Check sheet for the modelled part. Datum: model origin and axes. Units: mm. Face numbers are marked on the shaded views. A direction names the side the tool comes from. Round coordinates to 2 decimals unless told otherwise and drop trailing zeros. Loops run counter-clockwise (first coordinate to the right, second up) from the corner with the lowest first, then second, coordinate; pieces in that order, holes last. Notation, with made-up numbers: (18, 25.5) -> (32, 25.5) arc R3 ccw to (32, 29.5) -> close; hole circle Ø5 at (-10, 3). An arc over 180 degrees is marked (long way). One line per question, with ' | ' between items.
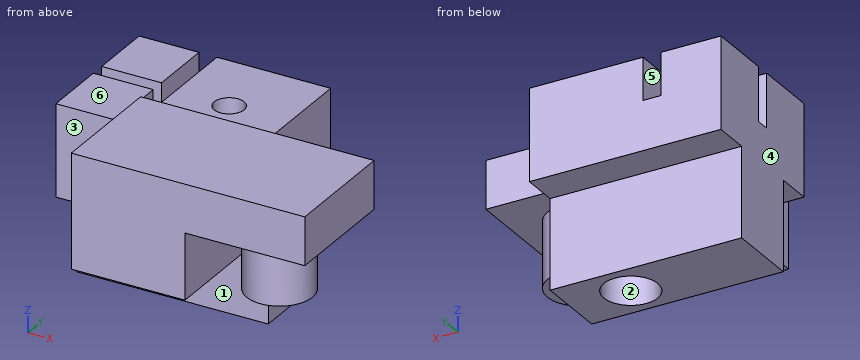
```python
from build123d import *

# Parameters (mm, degrees)
SKETCH_1_W          = 16
SKETCH_1_H          = 12
EXTRUDE_1_DEPTH     = 7.65
SKETCH_2_W          = 5
SKETCH_2_H          = 1.2
CUT_EXTRUDE_1_DEPTH = 4.5
SKETCH_3_R          = 7.15
CUT_EXTRUDE_2_DEPTH = 1.5
SKETCH_4_W          = 16
SKETCH_4_H          = 6
EXTRUDE_2_DEPTH     = 7.5
SKETCH_5_R          = 2.25
CUT_EXTRUDE_3_DEPTH = 7.5
SKETCH_6_R          = 1.25
CUT_EXTRUDE_4_DEPTH = 8.65
SKETCH_7_W          = 9.5
SKETCH_7_H          = 7.65
EXTRUDE_3_DEPTH     = 9
EXTRUDE_START       = -9.5
SKETCH_8_W          = 4
SKETCH_8_H          = 10
EXTRUDE_4_DEPTH     = 19.5
SKETCH_9_R          = 2.75
EXTRUDE_5_DEPTH     = 5.5


with BuildPart() as part:
    # Эскиз1 → Бобышка-Вытянуть1 (new body)
    with BuildSketch(Plane.XY):
        with Locations((-13.599693696, 25)):
            Rectangle(SKETCH_1_W, SKETCH_1_H)
    extrude(amount=EXTRUDE_1_DEPTH)

    # Эскиз2 → Вырез-Вытянуть1 (cut)
    with BuildSketch(Plane.XY.offset(7.65)):
        with Locations((-19.099693696, 25)):
            Rectangle(SKETCH_2_W, SKETCH_2_H)
    extrude(amount=-CUT_EXTRUDE_1_DEPTH, mode=Mode.SUBTRACT)

    # Эскиз3 → Вырез-Вытянуть2 (cut)
    with BuildSketch(Plane.ZY.offset(16.599693696)):
        with Locations((8, 25)):
            Circle(SKETCH_3_R)
    extrude(amount=-CUT_EXTRUDE_2_DEPTH, mode=Mode.SUBTRACT)

    # Эскиз4 → Бобышка-Вытянуть2 (add)
    with BuildSketch(Plane(origin=(0, 0, 0), x_dir=(-1, 0, 0), z_dir=(0, 0, -1))):
        with Locations((13.599693696, 25)):
            Rectangle(SKETCH_4_W, SKETCH_4_H)
    extrude(amount=EXTRUDE_2_DEPTH)

    # Эскиз5 → Вырез-Вытянуть3 (cut)
    with BuildSketch(Plane(origin=(0, 0, -7.5), x_dir=(-1, 0, 0), z_dir=(0, 0, -1))):
        with Locations((10.599693696, 25)):
            Circle(SKETCH_5_R)
    extrude(amount=-CUT_EXTRUDE_3_DEPTH, mode=Mode.SUBTRACT)

    # Эскиз6 → Вырез-Вытянуть4 (cut, through all)
    with BuildSketch(Plane(origin=(0, 0, 0), x_dir=(-1, 0, 0), z_dir=(0, 0, -1))):
        with Locations((10.599693696, 25)):
            Circle(SKETCH_6_R)
    extrude(amount=-CUT_EXTRUDE_4_DEPTH, mode=Mode.SUBTRACT)

    # Эскиз7 → Бобышка-Вытянуть3 (add)
    with BuildSketch(Plane.XZ.offset(-19)):
        with Locations((-10.349693696, 3.825)):
            Rectangle(SKETCH_7_W, SKETCH_7_H)
    extrude(amount=EXTRUDE_3_DEPTH)

    # Эскиз8 → Бобышка-Вытянуть4 (add)
    with BuildSketch(Plane(origin=(-5.599693696, 0, 0), x_dir=(0, 0, -1), z_dir=(1, 0, 0)).offset(EXTRUDE_START)):
        with Locations((-7.5, 15)):
            Rectangle(SKETCH_8_W, SKETCH_8_H)
    extrude(amount=EXTRUDE_4_DEPTH)

    # Эскиз9 → Бобышка-Вытянуть5 (add)
    with BuildSketch(Plane(origin=(0, 0, 5.5), x_dir=(-1, 0, 0), z_dir=(0, 0, -1))):
        with Locations((0.599693696, 15)):
            Circle(SKETCH_9_R)
    extrude(amount=EXTRUDE_5_DEPTH)


solid = part.part
```
(1) Sectioned sample at B-B, the plane z = 0.5. Record the cut outline in (x, y), and give its area (3 significant figures).
Answer:
outline: (-21.6, 19) -> (-15.1, 19) -> (-15.1, 10) -> (-5.6, 10) -> (-5.6, 31) -> (-21.6, 31) -> close; circle Ø5.5 at (-0.6, 15); hole circle Ø2.5 at (-10.6, 25) | area: 296 mm2
(2) Set-up check for the marked faces 1, 2 and 3: record each of +Z, -Z, +X, -X, +Y, -Y from which the full face is reachable in a straight line by a thin tool's end or side.
Answer:
face 1: -Z, +X, -X, -Y | face 2: -Z | face 3: +Z, -Z, -X, -Y
(3) Go/stop test with flat-tipped pins: pin 1 (3 mm diameter, centred on x = -16, y = 25, fed in from +Z); pin 2 (1.5 mm diameter, centred on x = -11.5, y = 29.5, fed in from -Z); pin 3 (3 mm diameter, centred on x = -18.5, z = 2, fed in from -Y); pin 4 (1 mm diameter, centred on y = 25.5, z = 3.5, fed in from -X). Record where each tip stops, or that it passes through.
Answer:
pin 1: stops at z = 7.65 | pin 2: stops at z = 0 | pin 3: stops at y = 19 | pin 4: stops at x = -21.6
(4) Sectioned sample at C-C, the plane x = -19. Record the cut outline in (y, z), and give its area (3 significant figures).
Answer:
outline: (19, 0) -> (22, 0) -> (22, -7.5) -> (28, -7.5) -> (28, 0) -> (31, 0) -> (31, 7.65) -> (25.6, 7.65) -> (25.6, 3.15) -> (24.4, 3.15) -> (24.4, 7.65) -> (19, 7.65) -> close | area: 131 mm2
(5) Sectioned sample at A-A, the plane z = 4.5. Record the cut outline in (x, y), and give its area (3 significant figures).
Answer:
outline: (-21.6, 19) -> (-16.6, 19) -> (-16.6, 24.4) -> (-21.6, 24.4) -> close; (-21.6, 25.6) -> (-16.6, 25.6) -> (-16.6, 31) -> (-21.6, 31) -> close; (-15.1, 10) -> (-5.6, 10) -> (-5.6, 31) -> (-15.1, 31) -> close; circle Ø5.5 at (-0.6, 15); hole circle Ø2.5 at (-10.6, 25) | area: 272 mm2
(6) Scan lines: probe 1 along X at (y, z) = (29.25, 7.5); probe 2 along Y at (x, z) = (-19.25, 2); probe 3 along Z at (x, y) = (-15, 17). Record each from-to range of solid material in increasing order.
Answer:
probe 1: x = -21.6 to -16.6, -15.1 to -5.6 | probe 2: y = 19 to 31 | probe 3: z = 0 to 9.5
(7) Sectioned sample at D-D, the plane y = 25. Record the cut outline in (x, z), and give its area (3 significant figures).
Answer:
outline: (-21.6, -7.5) -> (-12.85, -7.5) -> (-12.85, 0) -> (-11.85, 0) -> (-11.85, 7.65) -> (-15.1, 7.65) -> (-15.1, 0.85) -> (-16.6, 0.85) -> (-16.6, 3.15) -> (-21.6, 3.15) -> close; (-9.35, 0) -> (-8.35, 0) -> (-8.35, -7.5) -> (-5.6, -7.5) -> (-5.6, 7.65) -> (-9.35, 7.65) -> close | area: 157 mm2
(8) Mould release check, pull along X, two halves, no side actions. Record for the marked faces 4, 5 and 6: +X half, -X half, draft (parallel to the pull), parting line (faces both ways), or undercut.
Answer:
face 4: -X half | face 5: undercut | face 6: draft
